from build123d import *

# Parameters (mm, degrees)
F1_DEPTH = 359
F3_D     = 6
F4_D     = 6
F5_D     = 6
F6_D     = 6
F7_D     = 6
F7_DEPTH = 50


with BuildPart() as f1:
    # F0 (on Front) → F1 (new body)
    with BuildSketch(Plane.XZ):
        Polygon((-16.622992, 26.484536), (-21.622992, 26.484536), (-21.622992, -23.515464), (28.377008, -23.515464), (28.377008, -18.515464), (-16.622992, -18.515464), align=None)
    extrude(amount=F1_DEPTH)

    # F3 (through all)
    with Locations(Plane.YZ):
        with Locations((-334.5, 16.484536)):
            Hole(F3_D / 2)

    # F4 (through all)
    with Locations(Plane.YZ):
        with Locations((-24.5, 16.484536)):
            Hole(F4_D / 2)

    # F5 (through all)
    with Locations(Plane.YZ):
        with Locations((-299.5, 16.484536)):
            Hole(F5_D / 2)

    # F6 (through all)
    with Locations(Plane.YZ):
        with Locations((-59.5, 16.484536)):
            Hole(F6_D / 2)

    # F7
    with Locations(Plane.YZ):
        with Locations((-227, 17.484536), (-185, 17.484536)):
            Hole(F7_D / 2, depth=F7_DEPTH)


solid = f1.part
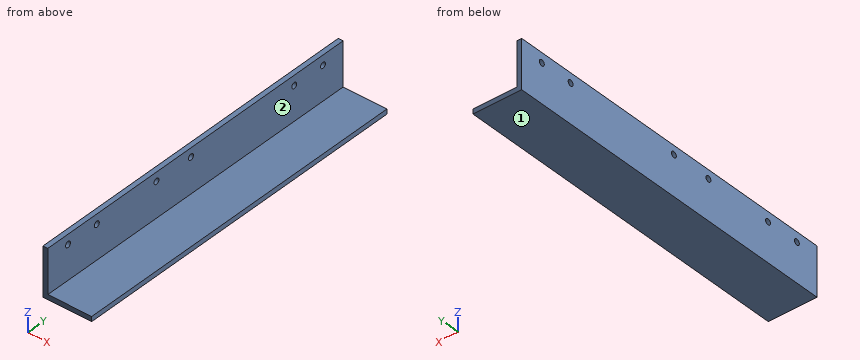
Build history of the part. All positions in model axes, mm. Face numbers are marked on the shaded views. A direction names the side the tool comes from. Give positions to 0.01 mm unless a question says otherwise; leave off trailing zeros. Order: outer loops, then holes, each group sorted by start corner. A loop starts at its lowest first (then second) coordinate and runs counter-clockwise, first axis right, second up. Notation, with made-up numbers: M 55.5,60.5 L 67.5,60.5 A35 cw 67.5,98.5 Z; hole C 54.5,20.25 d5. An arc over 180 degrees is marked long. Use one line per item in the form item = value.
1) Drop flat-ended pins along their axis: pin 1 (5.5 mm diameter, centred on y = -185, z = 17.48, fed in from -X); pin 2 (22.5 mm diameter, centred on x = -2, y = -249.5, fed in from +Z); pin 3 (7 mm diameter, centred on y = -334.5, z = 16.48, fed in from +X). Give the stop position or say it passes through.
Calculated:
pin_1 = through
pin_2 = -18.52
pin_3 = -16.62
2) Saw through at A-A (y = -24.5). Give the cut face in (x, z).
Calculated:
outline = M -21.62,-23.52 L 28.38,-23.52 L 28.38,-18.52 L -16.62,-18.52 L -16.62,13.48 L -21.62,13.48 Z; M -21.62,19.48 L -16.62,19.48 L -16.62,26.48 L -21.62,26.48 Z
3) Probe probe 1 along Z at (x, y) = (-18.65, -185); probe 2 along Z at (x, y) = (-20.4, -334.5); probe 3 along Z at (x, y) = (16, -178). List the from-to ranges inside material, lowest first.
Calculated:
probe_1 = -23.52 to 14.48, 20.48 to 26.48
probe_2 = -23.52 to 13.48, 19.48 to 26.48
probe_3 = -23.52 to -18.52
4) Saw through at C-C (x = 1). Give the cut face in (y, z), plus the area to 4 significant figures.
Calculated:
outline = M -359,-23.52 L 0,-23.52 L 0,-18.52 L -359,-18.52 Z
area = 1,795 mm2
5) Tool access for the marked faces 1 and 2: list every direction of +Z, -Z, +X, -X, +Y, -Y with a clear straight run to the whole face (end or side of a thin tool).
Calculated:
face_1 = -Z, +X, -X, +Y, -Y
face_2 = +Z, +X, +Y, -Y
6) Saw through at B-B (y = -192). Give the cut face in (x, z), plus the area to 3 significant figures.
Calculated:
outline = M -21.62,-23.52 L 28.38,-23.52 L 28.38,-18.52 L -16.62,-18.52 L -16.62,26.48 L -21.62,26.48 Z
area = 475 mm2
7) Saw through at D-D (z = 10). Give the cut face in (x, y), plus the area to 4 significant figures.
Calculated:
outline = M -21.62,-359 L -16.62,-359 L -16.62,0 L -21.62,0 Z
area = 1,795 mm2
